```python
from build123d import *

# Parameters (mm, degrees)
SKETCH1_W              = 0.3
SKETCH1_H              = 3
BOSS_EXTRUDE1_DEPTH    = 2.5
SKETCH1_3_W            = 0.3
SKETCH1_3_H            = 3
BOSS_EXTRUDE2_DEPTH    = 7.2
CUT_EXTRUDE1_START     = -2.45
CUT_EXTRUDE1_OUTLINE_R = 3
CUT_EXTRUDE1_DEPTH     = 8.2


# Read off the part's stored shape, not the designer's step: Cut-Extrude1
with BuildPart() as part:
    # Sketch1 → Boss-Extrude1 (new body)
    with BuildSketch(Plane(origin=(0, 0, 0), x_dir=(1, 0, 0), z_dir=(0, 1, 0))):
        with Locations((-5.175, -2.7)):
            Rectangle(SKETCH1_W, SKETCH1_H)
        with Locations((-4.875, -2.7)):
            Rectangle(SKETCH1_W, SKETCH1_H)
        with Locations((4.875, -2.7)):
            Rectangle(SKETCH1_W, SKETCH1_H)
        with Locations((5.175, -2.7)):
            Rectangle(SKETCH1_W, SKETCH1_H)
    extrude(amount=-BOSS_EXTRUDE1_DEPTH)

    # Sketch1_3 → Boss-Extrude2 (add)
    with BuildSketch(Plane(origin=(0, 0, 0), x_dir=(1, 0, 0), z_dir=(0, 1, 0))):
        Polygon((5.025, 5.75), (0, 5.75), (0, -5.75), (5.025, -5.75), (5.025, -4.2), (4.725, -4.2), (4.725, -1.2), (5.025, -1.2), align=None)
        Polygon((0, -5.75), (0, 5.75), (-5.025, 5.75), (-5.025, -1.2), (-4.725, -1.2), (-4.725, -4.2), (-5.025, -4.2), (-5.025, -5.75), align=None)
        with Locations((4.875, -2.7)):
            Rectangle(SKETCH1_3_W, SKETCH1_3_H)
        with Locations((-4.875, -2.7)):
            Rectangle(SKETCH1_3_W, SKETCH1_3_H)
    extrude(amount=BOSS_EXTRUDE2_DEPTH)

    # Cut-Extrude1 outline → Cut-Extrude1 (cut)
    with BuildSketch(Plane.XY.offset(CUT_EXTRUDE1_START)):
        with Locations((1.205, 3.5)):
            Circle(CUT_EXTRUDE1_OUTLINE_R)
    extrude(amount=CUT_EXTRUDE1_DEPTH, mode=Mode.SUBTRACT)


solid = part.part
```
Could you check a few things on this model? Use its own coordinates, in mm. A direction names the side the tool comes from. Round coordinates to 2 decimals unless told otherwise and drop trailing zeros. Write each loop counter-clockwise with the first axis right and the second up, starting at its lowest first coordinate (ties: lowest second). Pieces come first, ordered by that corner, then holes.
(1) Suppose I cut it at C-C on y = 3.5. Write out the boundary of the cut face in (x, z) (3 decimals), and give its area (3 significant figures).
Findings below:
outline: (-5.025, -5.75) - (5.025, -5.75) - (5.025, 5.75) - (4.205, 5.75) - (4.205, -2.45) - (-1.795, -2.45) - (-1.795, 5.75) - (-5.025, 5.75) - close
area: 66.4 mm2
(2) Suppose I cut it at A-A on z = 4. Write out the boundary of the cut face in (x, y) (3 decimals), and give its area (3 significant figures).
Findings below:
outline: (-5.325, -2.5) - (-4.725, -2.5) - (-4.725, 0) - (4.725, 0) - (4.725, -2.5) - (5.325, -2.5) - (5.325, 0) - (5.025, 0) - (5.025, 7.2) - (-5.025, 7.2) - (-5.025, 0) - (-5.325, 0) - close; hole circle Ø6 at (1.205, 3.5)
area: 47.1 mm2
(3) Suppose I cut it at B-B on y = -0.75. Write out the boundary of the cut face in (x, z) (3 decimals).
Findings below:
outline: (-5.325, 1.2) - (-4.725, 1.2) - (-4.725, 4.2) - (-5.325, 4.2) - close; (4.725, 1.2) - (5.325, 1.2) - (5.325, 4.2) - (4.725, 4.2) - close
(4) If I drill on probe 1 along Y at (x, z) = (1.25, 1.5); probe 2 along X at (y, z) = (4.5, -3.75) (3 decimals); probe 3 along Y at (x, z) = (4.5, 5.25), over which ranges is the centre line in solid material (lowest first)?
Findings below:
probe 1: y = 0 to 0.5, 6.5 to 7.2
probe 2: x = -5.025 to 5.025
probe 3: y = 0 to 7.2
(5) Which directions (+Z, -Z, +X, -X, +Y, -Y) give clear straight access to the entire face, cutting with the end or side of a thin tool? Please do faces 5 (the face through (1, 4, -2.45)), 6 (the face through (5.325, -1, 3)), 7 (the face through (0, 4, -5.75)), 8 (the face through (-5.025, 4, 0)), 9 (the face through (-4.725, -1, 3)).
Findings below:
face 5: +Z
face 6: +Z, -Z, +X, +Y, -Y
face 7: -Z, +X, -X, +Y, -Y
face 8: +Z, -Z, -X, +Y
face 9: +Z, -Z, -Y
(6) Suppose I cut it at D-D on x = 3.25. Write out the boundary of the cut face in (y, z).
Findings below:
outline: (0, -5.75) - (7.2, -5.75) - (7.2, 5.75) - (5.69, 5.75) - (5.69, -2.45) - (1.31, -2.45) - (1.31, 5.75) - (0, 5.75) - close
(7) For pin 1 (3.5 mm diameter, centred on y = 4.5, z = 2, fed in from +X) (3 decimals); pin 2 (3 mm diameter, centred on x = 1.5, z = -0.5, fed in from -Y); pin 3 (2 mm diameter, centred on y = 3.5, z = -1.5, fed in from -X) (3 decimals), each with a flat end and sliding along its axis, tell me the tip position at first contact or that it passes through.
Findings below:
pin 1: stops at x = 5.025
pin 2: stops at y = 0
pin 3: stops at x = -5.025
(8) Thinking about a two-plate mould opening in X: for faces 1 (the face through (4.066, 4.401, 1.593)), 2 (the face through (4.725, -1, 3)), 3 (the face through (5.025, 4, 0)), 4 (the face through (-2, 4, 5.75)), which applies, +X half, -X half, draft (parallel to the pull), parting line (faces both ways), or undercut?
Findings below:
face 1: undercut
face 2: undercut
face 3: +X half
face 4: draft
